from build123d import *

# Parameters (mm, degrees)
F0_R           = 55
F1_DEPTH       = 40
F2_DEPTH       = 300
F3_D           = 15.5
F5_D           = 17.5
F5_CBORE_D     = 31.5
F5_CBORE_DEPTH = 20
F7_DEPTH       = 200


with BuildPart() as f1:
    # F0 (on Front) → F1 (new body)
    with BuildSketch(Plane.XZ):
        with BuildLine():
            Line((-100, 40), (100, 40))
            Line((100, 40), (100, 200))
            ThreePointArc((100, 200), (0, 300), (-100, 200))
            Line((-100, 200), (-100, 40))
        make_face()
        with Locations((0, 200)):
            Circle(F0_R, mode=Mode.SUBTRACT)
    extrude(amount=F1_DEPTH)

    # F0 (on Front) → F2 (join)
    with BuildSketch(Plane.XZ):
        Polygon((-98.9183791646, 0), (0, 0), (100, 0), (100, 40), (-100, 40), (-100, 0), align=None)
    extrude(amount=F2_DEPTH)

    # F3 (through all)
    with Locations(Plane(origin=(0, 0, 0), x_dir=(1, 0, 0), z_dir=(0, 1, 0))):
        with Locations((0, -277), (-77, -200), (77, -200), (0, -123)):
            Hole(F3_D / 2)

    # F5 (through all)
    with Locations(Plane.XY.offset(40)):
        with Locations((-60, -140), (60, -140), (60, -260), (-60, -260)):
            CounterBoreHole(F5_D / 2, F5_CBORE_D / 2, F5_CBORE_DEPTH)

    # F6 (on face) → F7 (join)
    with BuildSketch(Plane.YZ.offset(100)):
        with BuildLine():
            ThreePointArc((-40, 50), (-42.9289321881, 42.9289321881), (-50, 40))
            Line((-50, 40), (-40, 40))
            Line((-40, 40), (-40, 50))
        make_face()
    extrude(amount=-F7_DEPTH)


solid = f1.part
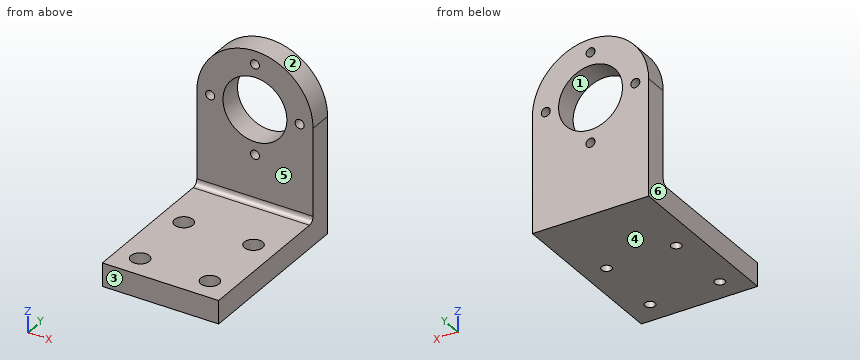
Model file for the job. Use its own axes, mm. Face numbers are marked on the shaded views. A direction names the side the tool comes from. Give positions to 0.01 mm unless a question says otherwise; leave off trailing zeros. Loops run counter-clockwise (first coordinate to the right, second up) from the corner with the lowest first, then second, coordinate; pieces in that order, holes last. Notation, with made-up numbers: (-14.75, -1.75) -> (27.25, -1.75) arc R30 cw to (27.25, 31.25) -> close; hole circle Ø5 at (74.25, 39). An arc over 180 degrees is marked (long way). Use a Markdown table: item, result. Add a question column.
(1) Slice it at A-A on z = 123. List the corners of the cut face in (x, y), and give its area (3 significant figures).
(2) Mould opens along Z. For the marked faces 1, 2, 3 and 4 say: +Z half, -Z half, draft (parallel to the pull), parting line (faces both ways), or undercut.
(3) Wall check: line 1 along Y through (x, z) = (-60, 25); line 2 along Y through (x, z) = (-60, 5); line 3 along Z through (x, y) = (0, -11). Give the ranges that are in metal, low to high.
(4) Slice it at C-C on x = 0. List the corners of the cut face in (y, z).
(5) Slice it at D-D on x = -31.5. List the corners of the cut face in (y, z), and give its area (3 significant figures).
(6) Drop flat-ended pins along their axis: pin 1 Ø25 at (x, y) = (60, -260) entering from -Z; pin 2 Ø16 at (x, y) = (52, -140.5) entering from +Z; pin 3 Ø12 at (x, z) = (-56.5, 115.5) entering from -Y; pin 4 Ø9.5 at (x, y) = (-56, -267) entering from +Z. Give the stop position or say it passes through.
(7) Tool access for the marked faces 5 and 6: list every direction of +Z, -Z, +X, -X, +Y, -Y with a clear straight run to the whole face (end or side of a thin tool).
(8) Slice it at B-B on y = -21. List the corners of the cut face in (x, z).
Filled sheet:
| question | item | result |
|---|---|---|
| 1 | outline | (-100, -40) -> (-7.75, -40) -> (-7.75, 0) -> (-100, 0) -> close; (7.75, -40) -> (100, -40) -> (100, 0) -> (7.75, 0) -> close |
| 1 | area | 7,380 mm2 |
| 2 | face 1 | undercut |
| 2 | face 2 | +Z half |
| 2 | face 3 | draft |
| 2 | face 4 | -Z half |
| 3 | line 1 | -300 to -275.75, -244.25 to -155.75, -124.25 to 0 |
| 3 | line 2 | -300 to -268.75, -251.25 to -148.75, -131.25 to 0 |
| 3 | line 3 | 0 to 115.25, 130.75 to 145, 255 to 269.25, 284.75 to 300 |
| 4 | outline | (-300, 0) -> (0, 0) -> (0, 115.25) -> (-40, 115.25) -> (-40, 50) arc R10 cw to (-50, 40) -> (-300, 40) -> close; (-40, 130.75) -> (0, 130.75) -> (0, 145) -> (-40, 145) -> close; (-40, 255) -> (0, 255) -> (0, 269.25) -> (-40, 269.25) -> close; (-40, 284.75) -> (0, 284.75) -> (0, 300) -> (-40, 300) -> close |
| 5 | outline | (-300, 0) -> (0, 0) -> (0, 154.91) -> (-40, 154.91) -> (-40, 50) arc R10 cw to (-50, 40) -> (-300, 40) -> close; (-40, 245.09) -> (0, 245.09) -> (0, 294.91) -> (-40, 294.91) -> close |
| 5 | area | 18,600 mm2 |
| 6 | pin 1 | z = 0 |
| 6 | pin 2 | z = 40 |
| 6 | pin 3 | y = -40 |
| 6 | pin 4 | z = 20 |
| 7 | face 5 | +Z, +X, -X, -Y |
| 7 | face 6 | +Z, -Z, -X, +Y, -Y |
| 8 | outline | (-100, 0) -> (100, 0) -> (100, 200) arc R100 ccw to (-100, 200) -> close; hole circle Ø15.5 at (-77, 200); hole circle Ø110 at (0, 200); hole circle Ø15.5 at (0, 123); hole circle Ø15.5 at (0, 277); hole circle Ø15.5 at (77, 200) |
